Here's how the part is built. I have some questions about the finished solid (model axes, mm). A direction names the side the tool comes from. Coordinates: 2 decimals unless noted, no trailing zeros. Write each loop counter-clockwise with the first axis right and the second up, starting at its lowest first coordinate (ties: lowest second). Pieces come first, ordered by that corner, then holes.
Autodesk Inventor part; units mm, degrees
ref_plane "Work Plane1" through (0, 0, 30) normal (0, 0, 1) x (1, 0, 0)
ref_plane "YZ Plane" through (0, 0, 0) normal (1, 0, 0) x (0, 1, 0)
ref_plane "XZ Plane" through (0, 0, 0) normal (0, 1, 0) x (-1, 0, 0)
sketch "Sketch1" plane through (0, 0, 0) normal (0, 0, 1) x (1, 0, 0)
  line L0 (0, 0) -> (50, 0)
  line L1 (50, 0) -> (50, 10)
  line L2 (50, 10) -> (0, 10)
  line L3 (0, 10) -> (0, 0)
  circle A0 centre (0, 10) radius 10
  point P0 (10, 10)
  dimension "d0" = 50
  dimension "d1" = 10
  dimension "d2" = 20
  dimension "d3" = 0
extrude "Extrusion1" add sketch "Sketch1" along normal blind 60 contours A0 L2 L1 L0
extrude "Extrusion2" add sketch "Sketch1" along normal blind 20 contours A0 L2 L3 | L3 L2 A0
ref_plane "Work Plane1" through (0, 0, 30) normal (0, 0, 1) x (1, 0, 0)
mirror "Mirror1" about plane through (0, 0, 30) normal (0, 0, 1) of "Extrusion2"
properties part number "left_hinge"
1. For pin 1 Ø12 at (y, z) = (11.5, 53.5) entering from -X; pin 2 Ø1.5 at (x, z) = (18, 49) entering from +Y; pin 3 Ø10 at (x, z) = (7.5, 40.5) entering from +Y; pin 4 Ø10 at (x, z) = (8, 22) entering from +Y, each with a flat end and sliding along its axis, tell me the tip position at first contact or that it passes through.
2. I want a section at A-A (y = 18.25). List the corners of the cut face in (x, z) for me.
3. I want a section at C-C (z = 37.5). List the corners of the cut face in (x, y) for me, then the cut area to 3 significant figures.
4. I want a section at B-B (x = -5.5). List the corners of the cut face in (y, z) for me.
5. I want a section at D-D (y = 4.5). List the corners of the cut face in (x, z) for me.
6. On a 3-axis mill with a long thin cutter (end or side, diameter ignored), from which of +Z, -Z, +X, -X, +Y, -Y can I reach the whole of each face in a straight line? I mean faces 1 (the face through (7.15, 3.01, 29.86)), 2 (the face through (50, 5, 30)), 3 (the face through (30, 10, 30)). Say none if no direction works.
7. Thinking about a two-plate mould opening in Z: for faces 4 (the face through (0, 10, 20)), 5 (the face through (13, 8, 60)), 6 (the face through (13, 8, 0)), 7 (the face through (-7.3, 16.834, 9.86)), which applies, pulls with the +Z half, pulls with the -Z half, needs draft (parallel to the pull), parting line crosses it, or undercut?
8. If I drill on line 1 (Z direction, x = -2.5, y = 14.5); line 2 (Y direction, x = 17.5, z = 41); line 3 (X direction, y = 15.5, z = 57.5), over which ranges is the centre line in solid material (lowest first)?
Response values:
1. pin 1: stops at x = -10
1. pin 2: stops at y = 10
1. pin 3: stops at y = 19.68
1. pin 4: stops at y = 19.4
2. outline: (-5.65, 0) - (5.65, 0) - (5.65, 20) - (-5.65, 20) - close; (-5.65, 40) - (5.65, 40) - (5.65, 60) - (-5.65, 60) - close
3. outline: (0, 0) - (50, 0) - (50, 10) - (10, 10) arc R10 cw to start
3. area: 421 mm2
4. outline: (1.65, 0) - (18.35, 0) - (18.35, 20) - (1.65, 20) - close; (1.65, 40) - (18.35, 40) - (18.35, 60) - (1.65, 60) - close
5. outline: (-8.35, 0) - (50, 0) - (50, 60) - (-8.35, 60) - (-8.35, 40) - (8.35, 40) - (8.35, 20) - (-8.35, 20) - close
6. face 1: -X, +Y
6. face 2: +Z, -Z, +X, +Y, -Y
6. face 3: +Z, -Z, +X, +Y
7. face 4: undercut
7. face 5: pulls with the +Z half
7. face 6: pulls with the -Z half
7. face 7: needs draft
8. line 1: z = 0 to 20, 40 to 60
8. line 2: y = 0 to 10
8. line 3: x = -8.35 to 8.35
